Design review of the part built by this model. Coordinates are the model's own, in mm. Coordinates: 2 decimals unless noted, no trailing zeros. Loops run counter-clockwise (first coordinate to the right, second up) from the corner with the lowest first, then second, coordinate; pieces in that order, holes last. Notation, with made-up numbers: (-0.5, -38.5) - (33.5, -38.5) arc R26 cw to (33.5, -5.5) - close; hole circle Ø1 at (25, 78.5). An arc over 180 degrees is marked (long way). Use one line per item in the form item = value. Start each with the question number.
(1) Clearance check with a flat-ended pin moving along its axis: pin 1 Ø11.5 at (x, z) = (-22.225, 76.2) entering from +Y. State where the tip first meets the part, or that it passes through.
(2) For L1, parallel to X at y = -7.5, z = 115; L2, parallel to Z at x = -56, y = -4.5; L3, parallel to X at y = -3.75, z = 110.5, list the stretches that pass through material, from the lowest coordinate up.
(3) Add section C-C (y = -3.5). Count the separate pieces of the cut face and the enclosed holes in it, plus the area to 3 significant figures.
(4) The part is to be moulded in two halves that separate along X. For faces 1 (the face through (-99.77, -12.52, 203.37)), 2 (the face through (-114.3, -13, 131)), 3 (the face through (0, -13, 131)), 4 (the face through (-39.553, -12.522, 145.104)), say which applies: pulls with the +X half, pulls with the -X half, needs draft (parallel to the pull), parting line crosses it, or undercut.
(5) Add section D-D (z = 38.1). State the section outline as (x, y) points (3 decimals).
(6) Add section B-B (z = 152.4). State the section outline as (x, y) points (3 decimals).
(7) Add section A-A (x = -57.15). State the section outline as (y, z) points.
```python
from build123d import *

# Parameters (mm, degrees)
F0_W     = 114.3
F0_H     = 266.7
F3_DEPTH = 25.4
F1_R     = 19.05
F4_DEPTH = 25.4
F2_R     = 6.35
F5_DEPTH = 25.4


with BuildPart() as f3:
    # F0 (on Front) → F3 (new body)
    with BuildSketch(Plane.XZ):
        with Locations((-57.15, 133.35)):
            Rectangle(F0_W, F0_H)
    extrude(amount=F3_DEPTH)

    # F1 (on face) → F4 (cut)
    with BuildSketch(Plane.XZ):
        with Locations((-85.725, 38.1)):
            Circle(F1_R)
        with Locations((-28.575, 38.1)):
            Circle(F1_R)
        with Locations((-57.15, 76.2)):
            Circle(F1_R)
        with Locations((-57.15, 152.4)):
            Circle(F1_R)
        with Locations((-28.575, 114.3)):
            Circle(F1_R)
        with Locations((-85.725, 114.3)):
            Circle(F1_R)
        with Locations((-28.575, 190.5)):
            Circle(F1_R)
        with Locations((-85.725, 190.5)):
            Circle(F1_R)
    extrude(amount=F4_DEPTH, mode=Mode.SUBTRACT)

    # F2 (on face) → F5 (cut)
    with BuildSketch(Plane.XZ):
        with BuildLine():
            ThreePointArc((-85.725, 76.2), (-96.565128, 80.690128), (-92.075, 69.85))
            ThreePointArc((-92.075, 69.85), (-87.584872, 71.709872), (-85.725, 76.2))
        make_face()
        with BuildLine():
            ThreePointArc((-15.875, 76.2), (-26.715128, 80.690128), (-22.225, 69.85))
            ThreePointArc((-22.225, 69.85), (-17.734872, 71.709872), (-15.875, 76.2))
        make_face()
        with Locations((-92.075, 152.4)):
            Circle(F2_R)
        with Locations((-22.225, 152.4)):
            Circle(F2_R)
    extrude(amount=F5_DEPTH, mode=Mode.SUBTRACT)


solid = f3.part
```
Computed values:
q1.pin_1 = through
q2.L1 = -114.3 to -104.76, -66.69 to -47.61, -9.54 to 0
q2.L2 = 0 to 57.18, 95.22 to 133.38, 171.42 to 266.7
q2.L3 = -114.3 to -104.39, -67.06 to -47.24, -9.91 to 0
q3.separate_pieces = 1
q3.enclosed_holes = 12
q3.area = 20,900 mm^2
q4.face_1 = undercut
q4.face_2 = pulls with the -X half
q4.face_3 = pulls with the +X half
q4.face_4 = undercut
q5.outline = (-114.3, -25.4) - (-104.775, -25.4) - (-104.775, 0) - (-114.3, 0) - close; (-66.675, -25.4) - (-47.625, -25.4) - (-47.625, 0) - (-66.675, 0) - close; (-9.525, -25.4) - (0, -25.4) - (0, 0) - (-9.525, 0) - close
q6.outline = (-114.3, -25.4) - (-98.425, -25.4) - (-98.425, 0) - (-114.3, 0) - close; (-85.725, -25.4) - (-76.2, -25.4) - (-76.2, 0) - (-85.725, 0) - close; (-38.1, -25.4) - (-28.575, -25.4) - (-28.575, 0) - (-38.1, 0) - close; (-15.875, -25.4) - (0, -25.4) - (0, 0) - (-15.875, 0) - close
q7.outline = (-25.4, 0) - (0, 0) - (0, 57.15) - (-25.4, 57.15) - close; (-25.4, 95.25) - (0, 95.25) - (0, 133.35) - (-25.4, 133.35) - close; (-25.4, 171.45) - (0, 171.45) - (0, 266.7) - (-25.4, 266.7) - close
